```python
from build123d import *

# Parameters (mm, degrees)
F1_DEPTH = 2.54
F3_DEPTH = 12.7
F4_R     = 2.54
F5_DEPTH = 25.4


# Not quite as in the source:
# - a feature names something its author has since deleted; it is built from what else it names


with BuildPart() as f1:
    # F0 (on Top) → F1 (new body)
    with BuildSketch(Plane.XY):
        Polygon((50.8, 63.5), (0, 63.5), (-50.8, 63.5), (-50.8, 50.8), (-63.5, 50.8), (-63.5, 0), (-63.5, -50.8), (-50.8, -50.8), (-50.8, -63.5), (0, -63.5), (50.8, -63.5), (50.8, -50.8), (63.5, -50.8), (63.5, 0), (63.5, 50.8), (50.8, 50.8), align=None)
    extrude(amount=F1_DEPTH)

    # F2 (on face) → F3 (join)
    with BuildSketch(Plane(origin=(0, 0, 0), x_dir=(1, 0, 0), z_dir=(0, 0, -1))):
        with BuildLine():
            Line((43.2105347984, -26.8235280358), (-43.2105347984, -26.8235280358))
            ThreePointArc((-43.2105347984, -26.8235280358), (-53.3766044151, -38.3837321185), (-42.2611118031, -49.0342304111))
            Line((-42.2611118031, -49.0342304111), (42.2611118031, -49.0342304111))
            ThreePointArc((42.2611118031, -49.0342304111), (53.3766044151, -38.3837321185), (43.2105347984, -26.8235280358))
        make_face()
    extrude(amount=F3_DEPTH)

    # F4 (on face) → F5 (cut)
    with BuildSketch(Plane.XY.offset(2.54)):
        with Locations((-44.45, 44.45)):
            Circle(F4_R)
        with Locations((-44.45, 31.75)):
            Circle(F4_R)
        with Locations((-31.75, 44.45)):
            Circle(F4_R)
        with Locations((-31.75, 31.75)):
            Circle(F4_R)
        with Locations((-19.05, 44.45)):
            Circle(F4_R)
        with Locations((-19.05, 31.75)):
            Circle(F4_R)
        with Locations((-6.35, 44.45)):
            Circle(F4_R)
        with Locations((-6.35, 31.75)):
            Circle(F4_R)
        with Locations((6.35, 44.45)):
            Circle(F4_R)
        with Locations((6.35, 31.75)):
            Circle(F4_R)
        with Locations((19.05, 44.45)):
            Circle(F4_R)
        with Locations((19.05, 31.75)):
            Circle(F4_R)
        with Locations((31.75, 44.45)):
            Circle(F4_R)
        with Locations((31.75, 31.75)):
            Circle(F4_R)
        with Locations((44.45, 44.45)):
            Circle(F4_R)
        with Locations((44.45, 31.75)):
            Circle(F4_R)
        with BuildLine():
            Line((44.45, 21.59), (-44.45, 21.59))
            ThreePointArc((-44.45, 21.59), (-46.99, 19.05), (-44.45, 16.51))
            Line((-44.45, 16.51), (44.45, 16.51))
            ThreePointArc((44.45, 16.51), (46.99, 19.05), (44.45, 21.59))
        make_face()
        with BuildLine():
            Line((44.45, 13.97), (-44.45, 13.97))
            ThreePointArc((-44.45, 13.97), (-46.99, 11.43), (-44.45, 8.89))
            Line((-44.45, 8.89), (44.45, 8.89))
            ThreePointArc((44.45, 8.89), (46.99, 11.43), (44.45, 13.97))
        make_face()
        with BuildLine():
            Line((44.45, 6.35), (-44.45, 6.35))
            ThreePointArc((-44.45, 6.35), (-46.99, 3.81), (-44.45, 1.27))
            Line((-44.45, 1.27), (44.45, 1.27))
            ThreePointArc((44.45, 1.27), (46.99, 3.81), (44.45, 6.35))
        make_face()
        with BuildLine():
            Line((44.45, -1.27), (-44.45, -1.27))
            ThreePointArc((-44.45, -1.27), (-46.99, -3.81), (-44.45, -6.35))
            Line((-44.45, -6.35), (44.45, -6.35))
            ThreePointArc((44.45, -6.35), (46.99, -3.81), (44.45, -1.27))
        make_face()
        with BuildLine():
            Line((44.45, -8.89), (-44.45, -8.89))
            ThreePointArc((-44.45, -8.89), (-46.99, -11.43), (-44.45, -13.97))
            Line((-44.45, -13.97), (44.45, -13.97))
            ThreePointArc((44.45, -13.97), (46.99, -11.43), (44.45, -8.89))
        make_face()
        with BuildLine():
            Line((44.45, -16.51), (-44.45, -16.51))
            ThreePointArc((-44.45, -16.51), (-46.99, -19.05), (-44.45, -21.59))
            Line((-44.45, -21.59), (44.45, -21.59))
            ThreePointArc((44.45, -21.59), (46.99, -19.05), (44.45, -16.51))
        make_face()
        with BuildLine():
            Line((44.45, -24.13), (-44.45, -24.13))
            ThreePointArc((-44.45, -24.13), (-46.99, -26.67), (-44.45, -29.21))
            Line((-44.45, -29.21), (44.45, -29.21))
            ThreePointArc((44.45, -29.21), (46.99, -26.67), (44.45, -24.13))
        make_face()
        with BuildLine():
            Line((44.45, -31.75), (-44.45, -31.75))
            ThreePointArc((-44.45, -31.75), (-46.99, -34.29), (-44.45, -36.83))
            Line((-44.45, -36.83), (44.45, -36.83))
            ThreePointArc((44.45, -36.83), (46.99, -34.29), (44.45, -31.75))
        make_face()
    extrude(amount=-F5_DEPTH, mode=Mode.SUBTRACT)


solid = f1.part
```
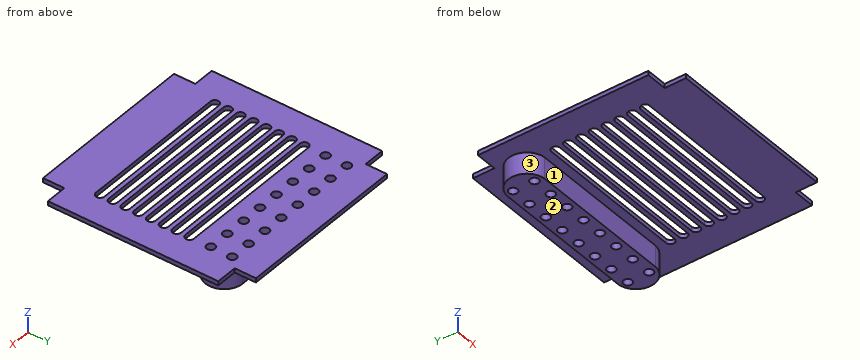
Design review of the part built by this model. Coordinates are the model's own, in mm. Face numbers are marked on the shaded views. A direction names the side the tool comes from. Give positions to 0.01 mm unless a question says otherwise; leave off trailing zeros. Write each loop counter-clockwise with the first axis right and the second up, starting at its lowest first coordinate (ties: lowest second). Pieces come first, ordered by that corner, then holes. Notation, with made-up numbers: (18.5, -32.5) - (76.5, -32.5) arc R19 ccw to (76.5, -4.5) - close; hole circle Ø6 at (80.5, 67). An arc over 180 degrees is marked (long way). Return JSON: item names as keys, results as strings. Group by question number.
(1) Machinability: for the marked faces 1, 2 and 3, which of the approach directions +Z, -Z, +X, -X, +Y, -Y give a long, thin tool a straight path to every point of the face, cutting with its end or side? Answer none if there is none.
(2) To check wall thickness, follow probe 1 along Y at (x, z) = (-31.75, -1.25); probe 2 along Y at (x, z) = (44.45, -3); probe 3 along Y at (x, z) = (-24, -6.5). State the ranges of each line that lie inside material, in increasing order.
(3) We need section C-C, the plane y = -54.5. Give the boundary of the cut face in (x, z).
(4) Insertion check: pin 1 (1 mm diameter, centred on y = 37, z = -5, fed in from -X); pin 2 (8 mm diameter, centred on x = -6.35, y = 31.75, fed in from -Z); pin 3 (1.5 mm diameter, centred on x = 1.5, z = -6, fed in from +Y); pin 4 (3 mm diameter, centred on x = 59.5, z = 1, fed in from +Y). Each pin has a flat end and moves straight along its axis. Give the tip position at first contact, or say it passes through.
(5) We need section A-A, the plane y = -11.43. Give the boundary of the cut face in (x, z), then the cut area to 3 significant figures.
(6) We need section D-D, the plane x = -49. Give the boundary of the cut face in (y, z), then the cut area to 3 significant figures.
(7) We need section B-B, the plane x = 19.05. Give the number of separate pieces and of enclosed holes in the cut face, then the cut area to 3 significant figures.
Reported:
{
 "1": {"face 1": "-Z, +X, -X, -Y", "face 2": "-Z, +X, -X, +Y, -Y", "face 3": "-Z, -X"},
 "2": {"probe 1": "y = 26.82 to 29.21, 34.29 to 41.91, 46.99 to 49.03", "probe 2": "y = 27 to 29.21, 34.29 to 41.91, 46.99 to 48.82", "probe 3": "y = 26.82 to 49.03"},
 "3": {"outline": "(-50.8, 0) - (50.8, 0) - (50.8, 2.54) - (-50.8, 2.54) - close"},
 "4": {"pin 1": "stops at x = -53.38", "pin 2": "stops at z = -12.7", "pin 3": "stops at y = 49.03", "pin 4": "stops at y = 50.8"},
 "5": {"outline": "(-63.5, 0) - (-46.99, 0) - (-46.99, 2.54) - (-63.5, 2.54) - close; (46.99, 0) - (63.5, 0) - (63.5, 2.54) - (46.99, 2.54) - close", "area": "83.9 mm2"},
 "6": {"outline": "(-63.5, 0) - (29.06, 0) - (29.06, -12.7) - (46.76, -12.7) - (46.76, 0) - (63.5, 0) - (63.5, 2.54) - (-63.5, 2.54) - close", "area": "547 mm2"},
 "7": {"separate pieces": "11", "enclosed holes": "0", "area": "347 mm2"}
}
